The model under review builds one solid part; all positions refer to its coordinate system, in mm. A direction names the side the tool comes from. Coordinates: 2 decimals unless noted, no trailing zeros. Order: outer loops, then holes, each group sorted by start corner. A loop starts at its lowest first (then second) coordinate and runs counter-clockwise, first axis right, second up. Notation, with made-up numbers: M -36.5,-28 L 5.5,-28 A21 ccw 5.5,-23 Z; hole C 4,61 d1. An arc over 180 degrees is marked long. One line per item, written item: value.
```python
from build123d import *

# Parameters (mm, degrees)
F0_W     = 85
F0_H     = 6.6378710747
F0_H_2   = 7.9
F1_DEPTH = 4
F2_DEPTH = 2.5
F4_D     = 4.4
F4_DEPTH = 25
F4_TIP   = 1.3218933619
F6_DEPTH = 4
F7_D     = 3.3
F7_DEPTH = 25
F7_TIP   = 0.9914200214
F8_R     = 2


with BuildPart() as f1:
    # F0 (on Top) → F1 (new body)
    with BuildSketch(Plane.XY):
        with Locations((0, 7.2689355373)):
            Rectangle(F0_W, F0_H)
        Rectangle(F0_W, F0_H_2)
        with Locations((0, -7.2689355373)):
            Rectangle(F0_W, F0_H)
    extrude(amount=-F1_DEPTH)

    # F0 (on Top) → F2 (join)
    with BuildSketch(Plane.XY):
        with Locations((0, 7.2689355373)):
            Rectangle(F0_W, F0_H)
        with Locations((0, -7.2689355373)):
            Rectangle(F0_W, F0_H)
    extrude(amount=F2_DEPTH)

    # F4
    with Locations(Plane.XY.offset(2.5)):
        with Locations((-37.9123874009, 6.7939041182), (-37.9123874009, -6.7939041182), (-26.9123874009, 6.7939041182), (-26.9123874009, -6.7939041182), (-15.9123874009, 6.7939041182), (-15.9123874009, -6.7939041182), (-4.9123874009, 6.7939041182), (-4.9123874009, -6.7939041182), (6.0876125991, 6.7939041182), (6.0876125991, -6.7939041182), (17.0876125991, -6.7939041182), (17.0876125991, 6.7939041182), (28.0876125991, 6.7939041182), (28.0876125991, -6.7939041182), (39.0876125991, -6.7939041182), (39.0876125991, 6.7939041182)):
            Hole(F4_D / 2, depth=F4_DEPTH)
            with Locations((0, 0, -(F4_DEPTH + F4_TIP / 2))):  # 118° drill point
                Cone(0, F4_D / 2, F4_TIP, mode=Mode.SUBTRACT)

    # F5 (on Top) → F6 (join)
    with BuildSketch(Plane.XY):
        Polygon((51.1790141463, 10.5878710747), (42.4563325942, 10.5878710747), (42.5, 0), (51.1790141463, 0), align=None)
    extrude(amount=-F6_DEPTH)

    # F7
    with Locations(Plane.XY):
        with Locations((47.7968230844, 5.1023042761)):
            Hole(F7_D / 2, depth=F7_DEPTH)
            with Locations((0, 0, -(F7_DEPTH + F7_TIP / 2))):  # 118° drill point
                Cone(0, F7_D / 2, F7_TIP, mode=Mode.SUBTRACT)

    # F8
    f8_edges = [f1.edges().sort_by_distance(p)[0] for p in [
        (-42.5, 10.587871, -0.75),
        (-42.5, -10.587871, -0.75),
        (51.179014, 10.587871, -2),
        (51.179014, 0, -2),
        (42.5, -10.587871, -0.75),
        (42.5, 0, -2),
    ]]
    fillet(f8_edges, radius=F8_R)


solid = f1.part
```
(1) We need section B-B, the plane z = -1.25. Count the separate pieces of the cut face and the enclosed holes in it, plus the area to 3 significant figures.
Geometry results:
separate pieces: 1
enclosed holes: 17
area: 1,640 mm2
(2) Mouldability with a two-part tool opening along Y and no side actions: class faces 3 (the cylindrical face through (43.07, -0.6, -2.03)), 4 (the cylindrical face through (50.578, 10.018, -2.028)), 5 (the cylindrical face through (7.833, -8.133, -0.796)) as +Y half, -Y half, draft (parallel to the pull), parting line (faces both ways), or undercut.
Geometry results:
face 3: -Y half
face 4: +Y half
face 5: undercut
(3) We need section A-A, the plane x = -21.5. State the section outline as (y, z) points, plus the area to 3 significant figures.
Geometry results:
outline: M -10.59,-4 L 10.59,-4 L 10.59,2.5 L 3.95,2.5 L 3.95,0 L -3.95,0 L -3.95,2.5 L -10.59,2.5 Z
area: 118 mm2
(4) Tool access review of faces 1 (the flat face through (42.5, -5, -1)), 2 (the flat face through (-1, -10.588, -1)): name each direction out of +Z, -Z, +X, -X, +Y, -Y from which nothing blocks a thin tool from reaching the whole face with its end or side.
Geometry results:
face 1: +Z, -Z, +X, -Y
face 2: +Z, -Z, +X, -X, -Y
(5) For L1, parallel to Y at x = 25, z = 1; L2, parallel to Y at x = -4, z = 1; L3, parallel to Z at x = -20.5, y = -3, list the stretches that pass through material, from the lowest coordinate up.
Geometry results:
L1: y = -10.59 to -3.95, 3.95 to 10.59
L2: y = -10.59 to -8.8, -4.79 to -3.95, 3.95 to 4.79, 8.8 to 10.59
L3: z = -4 to 0
(6) Insertion check: pin 1 Ø2 at (y, z) = (-5.5, -1) entering from +X; pin 2 Ø3.5 at (x, y) = (39.09, 6.79) entering from +Z; pin 3 Ø4 at (x, y) = (47.8, 5.1) entering from +Z; pin 4 Ø3 at (x, z) = (46.5, -1) entering from -Y. Each pin has a flat end and moves straight along its axis. Give the tip position at first contact, or say it passes through.
Geometry results:
pin 1: stops at x = 42.5
pin 2: passes through
pin 3: stops at z = 0
pin 4: stops at y = 0
